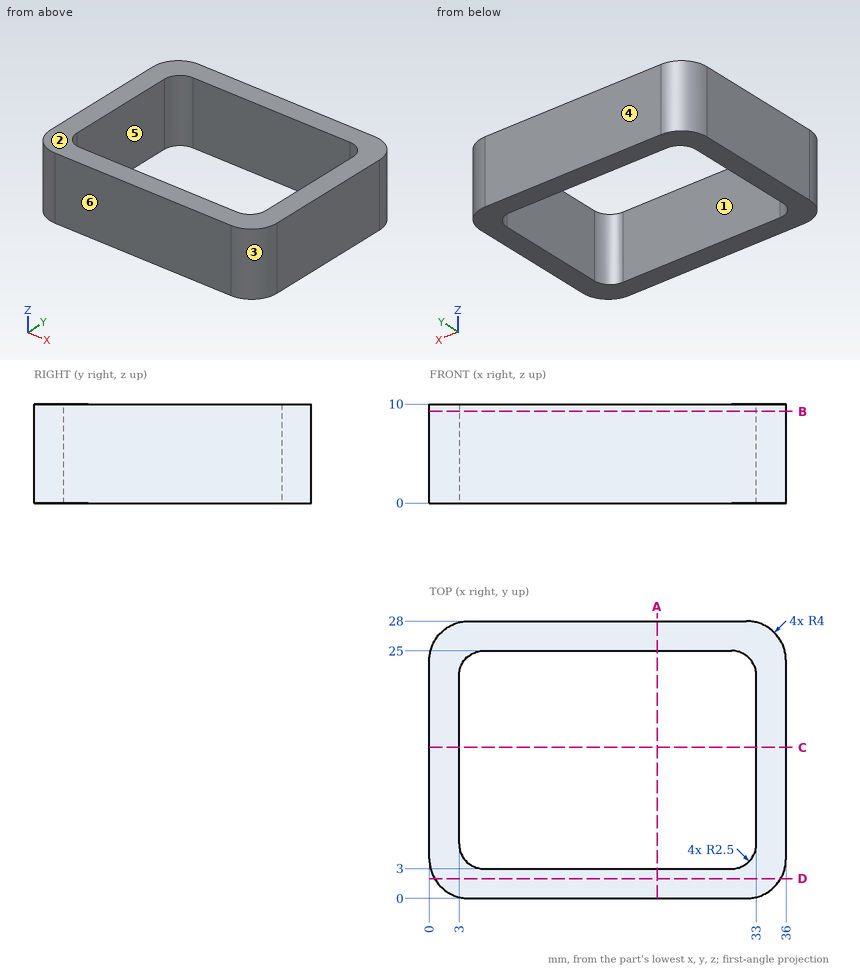
Verification items for this drawing (mm, ordinates from the low corner). A direction names the side the tool comes from. Coordinates: 2 decimals unless noted, no trailing zeros. Order: outer loops, then holes, each group sorted by start corner. A loop starts at its lowest first (then second) coordinate and runs counter-clockwise, first axis right, second up. Notation, with made-up numbers: (30.5, -13) - (84.5, -13) arc R13 ccw to (84.5, 0) - close; hole circle Ø5 at (11, -4.75). An arc over 180 degrees is marked (long way). Answer as a JSON object with one key per item and string values. Group by question number.
Item 1: Sectioned sample at A-A, the plane x = 23. Record the cut outline in (y, z), and give its area (3 significant figures).
Item 2: Depth check by flat-ended pin: pin 1 Ø1.5 at (y, z) = (25, 3) entering from -X. Enter the tip coordinate at first touch or a pass-through.
Item 3: Sectioned sample at C-C, the plane y = 15.25. Record the cut outline in (x, z), and give its area (3 significant figures).
Item 4: Sectioned sample at D-D, the plane y = 2. Record the cut outline in (x, z).
Item 5: Draft check along Y on the marked faces 1, 2, 3 and 4. Enter one of: +Y half, -Y half, draft (parallel to the pull), parting line (faces both ways), or undercut.
Item 6: Sectioned sample at B-B, the plane z = 9.25. Record the cut outline in (x, y), and give its area (3 significant figures).
Item 7: Tool access check on the marked faces 5 and 6. Record the directions out of +Z, -Z, +X, -X, +Y, -Y that give a thin tool (end or side, any length) a straight path to the whole face; none if there is none.
Item 8: Scan lines: probe 1 along Y at (x, z) = (11.5, 0.5); probe 2 along X at (y, z) = (19.25, 6.5); probe 3 along X at (y, z) = (4, 7.5). Record each from-to range of solid material in increasing order.
Resolved:
{
 "1": {"outline": "(0, 0) - (3, 0) - (3, 10) - (0, 10) - close; (25, 0) - (28, 0) - (28, 10) - (25, 10) - close", "area": "60.0 mm^2"},
 "2": {"pin 1": "x = 0.01"},
 "3": {"outline": "(0, 0) - (3, 0) - (3, 10) - (0, 10) - close; (33, 0) - (36, 0) - (36, 10) - (33, 10) - close", "area": "60.0 mm^2"},
 "4": {"outline": "(0.54, 0) - (35.46, 0) - (35.46, 10) - (0.54, 10) - close"},
 "5": {"face 1": "undercut", "face 2": "draft", "face 3": "-Y half", "face 4": "+Y half"},
 "6": {"outline": "(0, 4) arc R4 ccw to (4, 0) - (32, 0) arc R4 ccw to (36, 4) - (36, 24) arc R4 ccw to (32, 28) - (4, 28) arc R4 ccw to (0, 24) - close; hole (3, 5.5) arc R2.5 ccw to (5.5, 3) - (30.5, 3) arc R2.5 ccw to (33, 5.5) - (33, 22.5) arc R2.5 ccw to (30.5, 25) - (5.5, 25) arc R2.5 ccw to (3, 22.5) - close", "area": "340 mm^2"},
 "7": {"face 5": "+Z, -Z", "face 6": "+Z, -Z, +X, -X, -Y"},
 "8": {"probe 1": "0 to 3, 25 to 28", "probe 2": "0 to 3, 33 to 36", "probe 3": "0 to 3.5, 32.5 to 36"}
}
